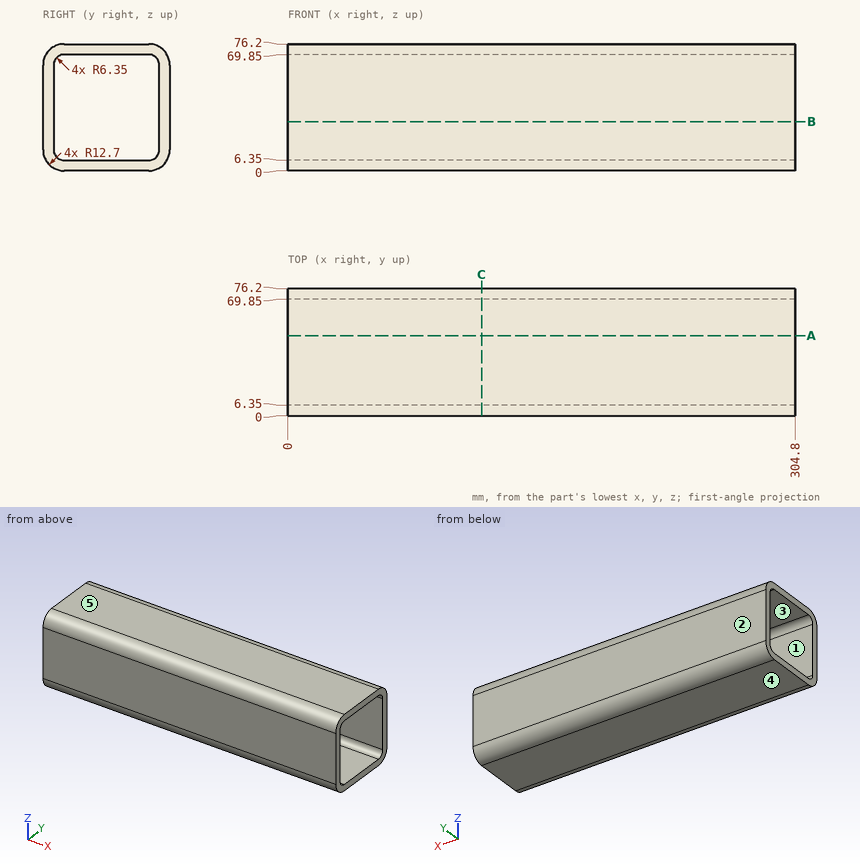
For this review, use the dimensioned drawing (mm, ordinates from the lowest corner) and the shaded views. A direction names the side the tool comes from. Round coordinates to 2 decimals unless told otherwise and drop trailing zeros. Write each loop counter-clockwise with the first axis right and the second up, starting at its lowest first coordinate (ties: lowest second). Pieces come first, ordered by that corner, then holes. Notation, with made-up numbers: M 27.25,-24 L 37.25,-24 A30 ccw 37.25,-1 Z; hole C 76.25,-21 d9. An arc over 180 degrees is marked long. Use CSV: the item, a comma, the result in double quotes. Start each with the question number.
(1) Tool access review of the marked faces 1 and 2: name each direction out of +Z, -Z, +X, -X, +Y, -Y from which nothing blocks a thin tool from reaching the whole face with its end or side.
(2) We need section A-A, the plane y = 48. State the section outline as (x, z) points, then the cut area to 3 significant figures.
(3) The part is to be moulded in two halves that separate along Z. For the marked faces 3, 4 and 5, say which applies: +Z half, -Z half, draft (parallel to the pull), parting line (faces both ways), or undercut.
(4) We need section C-C, the plane x = 116.5. State the section outline as (y, z) points, then the cut area to 3 significant figures.
(5) For line 1 along Z through (x, y) = (253, 22); line 2 along Z through (x, y) = (40, 66), list the stretches that pass through material, from the lowest coordinate up.
Findings:
1,face 1,"+X, -X"
1,face 2,"+Z, -Z, +X, -X, +Y"
2,outline,"M 0,0 L 304.8,0 L 304.8,6.35 L 0,6.35 Z; M 0,69.85 L 304.8,69.85 L 304.8,76.2 L 0,76.2 Z"
2,area,"3,870 mm^2"
3,face 3,"undercut"
3,face 4,"-Z half"
3,face 5,"+Z half"
4,outline,"M 0,12.7 A12.7 ccw 12.7,0 L 63.5,0 A12.7 ccw 76.2,12.7 L 76.2,63.5 A12.7 ccw 63.5,76.2 L 12.7,76.2 A12.7 ccw 0,63.5 Z; hole M 6.35,12.7 A6.35 ccw 12.7,6.35 L 63.5,6.35 A6.35 ccw 69.85,12.7 L 69.85,63.5 A6.35 ccw 63.5,69.85 L 12.7,69.85 A6.35 ccw 6.35,63.5 Z"
4,area,"1,670 mm^2"
5,line 1,"0 to 6.35, 69.85 to 76.2"
5,line 2,"0.25 to 6.86, 69.34 to 75.95"
